The figure shows three views and two pictorial views of one solid part (mm, origin at its lowest corner). Answer the questions. Coordinates: 2 decimals unless noted, no trailing zeros. Write each loop counter-clockwise with the first axis right and the second up, starting at its lowest first coordinate (ties: lowest second). Pieces come first, ordered by that corner, then holes.
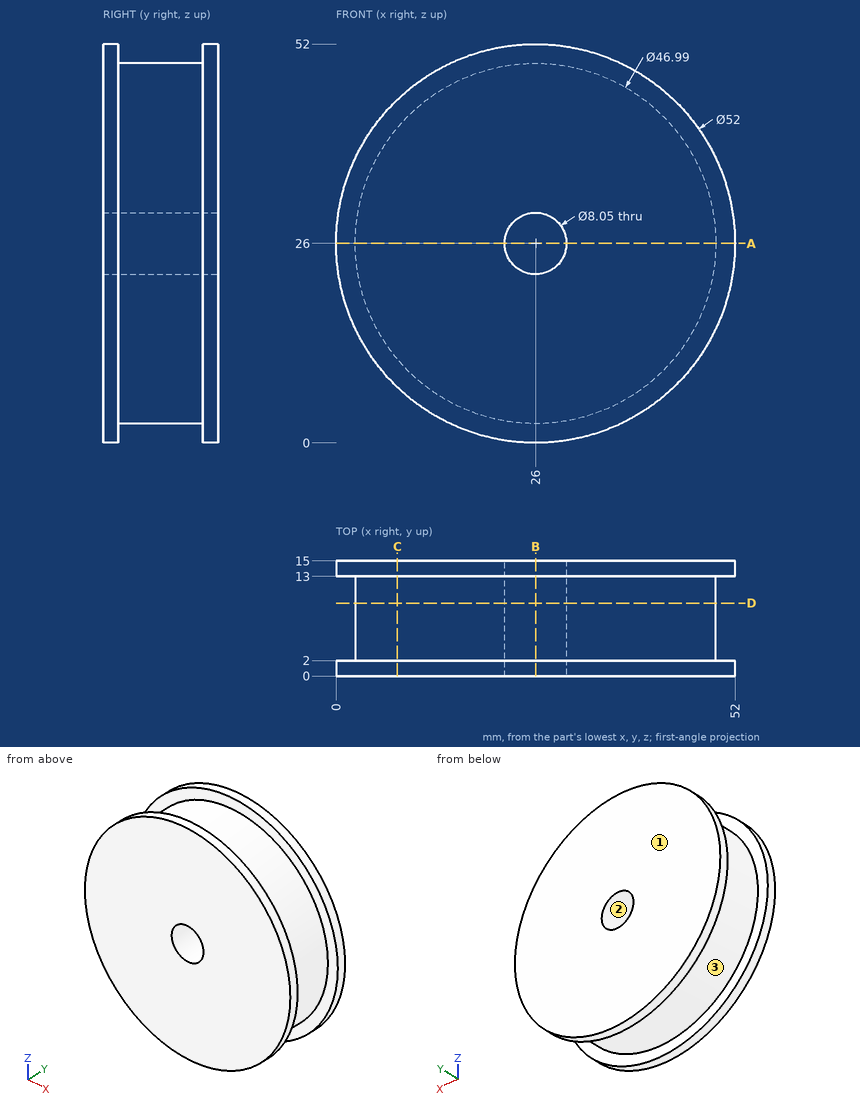
1. Section D-D on y = 9.5 is taken. Give the vertices of the cut face in (x, z) (3 decimals).
Results found:
outline: circle Ø46.99 at (26, 26); hole circle Ø8.05 at (26, 26)
2. For a pull along Z with two mould halves and no side action, classify the marked faces 1, 2 and 3 as pulls with the +Z half, pulls with the -Z half, needs draft (parallel to the pull), parting line crosses it, or undercut.
Results found:
face 1: needs draft
face 2: undercut
face 3: parting line crosses it
3. Section C-C on x = 8 is taken. Give the vertices of the cut face in (y, z), then the cut area to 3 significant figures.
Results found:
outline: (0, 7.24) - (2, 7.24) - (2, 10.9) - (13, 10.9) - (13, 7.24) - (15, 7.24) - (15, 44.76) - (13, 44.76) - (13, 41.1) - (2, 41.1) - (2, 44.76) - (0, 44.76) - close
area: 482 mm2
4. Find the intervals of material crossed by L1, parallel to Z at x = 26, y = 6 (3 decimals); L2, parallel to Y at x = 42.5, z = 6.5, in increasing order.
Results found:
L1: z = 2.505 to 21.975, 30.025 to 49.495
L2: y = 0 to 2, 13 to 15
5. Flat-ended cylindrical pins translate along their axes: P1, Ø2, axis at x = 27.5, y = 13, coming from the +Z side; P2, Ø3, axis at y = 5.5, z = 13.5, coming from the -X side; P3, Ø1, axis at x = 25, y = 2, coming from the -Z side. Find the tip coordinate at first contact, or state that the pin passes through.
Results found:
P1: stops at z = 52
P2: stops at x = 5.24
P3: stops at z = 0
6. Section A-A on z = 26 is taken. Give the vertices of the cut face in (x, y) (3 decimals).
Results found:
outline: (0, 0) - (21.975, 0) - (21.975, 15) - (0, 15) - (0, 13) - (2.505, 13) - (2.505, 2) - (0, 2) - close; (30.025, 0) - (52, 0) - (52, 2) - (49.495, 2) - (49.495, 13) - (52, 13) - (52, 15) - (30.025, 15) - close
7. Section B-B on x = 26 is taken. Give the vertices of the cut face in (y, z) (3 decimals), then the cut area to 3 significant figures.
Results found:
outline: (0, 0) - (2, 0) - (2, 2.505) - (13, 2.505) - (13, 0) - (15, 0) - (15, 21.975) - (0, 21.975) - close; (0, 30.025) - (15, 30.025) - (15, 52) - (13, 52) - (13, 49.495) - (2, 49.495) - (2, 52) - (0, 52) - close
area: 604 mm2
